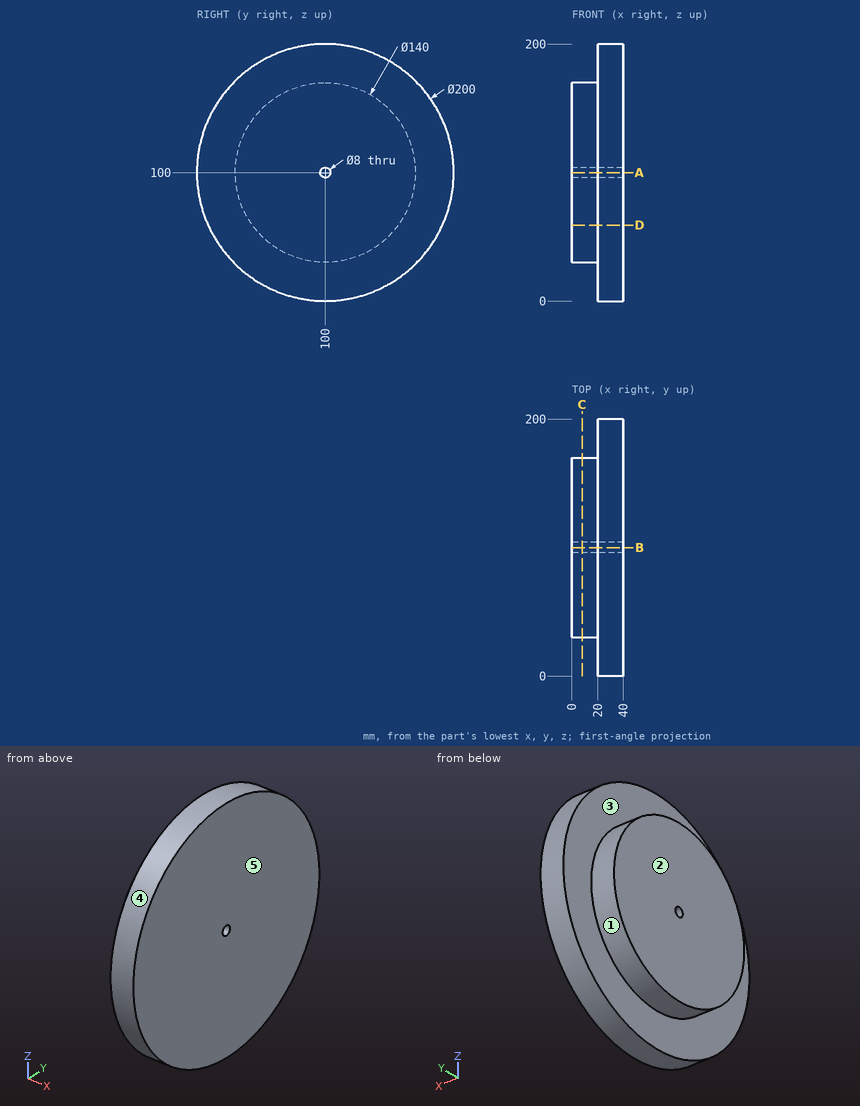
Check sheet for the drawn part. Datum: minimum x, y, z corner. Units: mm. A direction names the side the tool comes from. Round coordinates to 2 decimals unless told otherwise and drop trailing zeros. Loops run counter-clockwise (first coordinate to the right, second up) from the corner with the lowest first, then second, coordinate; pieces in that order, holes last.
Item 1: Thickness scan on line 1 (Y direction, x = 22, z = 100); line 2 (X direction, y = 20.5, z = 108); line 3 (Z direction, x = 12.5, y = 99). Record the ranges inside material, lowest first.
Item 2: Gauge pin test, flat ends, axial feed: pin 1 (1.5 mm diameter, centred on y = 131, z = 171.5, fed in from -X); pin 2 (10 mm diameter, centred on x = 33.5, y = 132, fed in from -Z); pin 3 (1 mm diameter, centred on x = 22.5, y = 179, fed in from +Z); pin 4 (6.5 mm diameter, centred on y = 100, z = 100, fed in from +X). Record the tip position at first contact, or that the pin passes through.
Item 3: Cross-section at D-D on z = 59. Record the boundary of the cut face in (x, y).
Item 4: Access from +Z, -Z, +X, -X, +Y, -Y to the whole of each face (thin tool, end or side, straight path). Record for the marked faces 1 and 2.
Item 5: Cross-section at A-A on z = 100. Record the boundary of the cut face in (x, y), then the cut area to 3 significant figures.
Item 6: Cross-section at C-C on x = 8. Record the boundary of the cut face in (y, z).
Item 7: Mould release check, pull along X, two halves, no side actions. Record for the marked faces 3, 4 and 5: pulls with the +X half, pulls with the -X half, needs draft (parallel to the pull), parting line crosses it, or undercut.
Answer sheet:
1. line 1: y = 0 to 96, 104 to 200
1. line 2: x = 20 to 40
1. line 3: z = 30.01 to 96.13, 103.87 to 169.99
2. pin 1: stops at x = 20
2. pin 2: stops at z = 3.71
2. pin 3: stops at z = 161.95
2. pin 4: passes through
3. outline: (0, 43.26) - (20, 43.26) - (20, 8.79) - (40, 8.79) - (40, 191.21) - (20, 191.21) - (20, 156.74) - (0, 156.74) - close
4. face 1: -X
4. face 2: +Z, -Z, -X, +Y, -Y
5. outline: (0, 30) - (20, 30) - (20, 0) - (40, 0) - (40, 96) - (0, 96) - close; (0, 104) - (40, 104) - (40, 200) - (20, 200) - (20, 170) - (0, 170) - close
5. area: 6,480 mm2
6. outline: circle Ø140 at (100, 100); hole circle Ø8 at (100, 100)
7. face 3: pulls with the -X half
7. face 4: needs draft
7. face 5: pulls with the +X half
